```python
from build123d import *

# Parameters (mm, degrees)
F0_R     = 14.2875
F0_R_2   = 3.373438
F1_DEPTH = 2.286


with BuildPart() as f1:
    # F0 (on Front) → F1 (new body)
    with BuildSketch(Plane.XZ):
        with BuildLine():
            ThreePointArc((-34.573266, -67.66252), (-26.367008, -66.963304), (-18.815872, -63.675156))
            Line((-18.815872, -63.675156), (136.129614, 36.414264))
            ThreePointArc((136.129614, 36.414264), (146.710231, 64.934436), (122.34748, 83.14998))
            Line((122.34748, 83.14998), (37.837742, 83.14998))
            ThreePointArc((37.837742, 83.14998), (27.550148, 85.3266), (19.025718, 91.483412))
            Line((19.025718, 91.483412), (-13.74376, 116.798291))
            ThreePointArc((-13.74376, 116.798291), (-32.877689, 121.840327), (-49.823331, 111.623939))
            Line((-49.823331, 111.623939), (-138.293377, -10.186806))
            ThreePointArc((-138.293377, -10.186806), (-141.899369, -17.266125), (-143.141887, -25.113168))
            Line((-143.141887, -25.113168), (-143.141887, -42.26252))
            ThreePointArc((-143.141887, -42.26252), (-135.7024, -60.223032), (-117.741887, -67.66252))
            Line((-117.741887, -67.66252), (-34.573266, -67.66252))
        make_face()
        with Locations((-20.212744, -35.91252)):
            Circle(F0_R, mode=Mode.SUBTRACT)
        Polygon((-75.897325, -20.576264), (-88.5972, -20.519901), (-94.898326, -9.493306), (-88.499577, 1.476927), (-75.799702, 1.420565), (-69.498576, -9.606031), align=None, mode=Mode.SUBTRACT)
        Polygon((-75.839717, 7.770723), (-88.539592, 7.827085), (-94.840718, 18.853681), (-88.441969, 29.823914), (-75.742094, 29.767551), (-69.440968, 18.740956), align=None, mode=Mode.SUBTRACT)
        Polygon((-48.344767, -5.516115), (-61.044642, -5.459752), (-67.345768, 5.566844), (-60.947019, 16.537077), (-48.247144, 16.480714), (-41.946018, 5.454118), align=None, mode=Mode.SUBTRACT)
        Polygon((6.38129, -3.277528), (-6.318585, -3.221165), (-12.619711, 7.80543), (-6.220962, 18.775663), (6.478913, 18.719301), (12.780039, 7.692705), align=None, mode=Mode.SUBTRACT)
        Polygon((-19.443963, 11.747547), (-32.143838, 11.80391), (-38.444964, 22.830506), (-32.046215, 33.800739), (-19.34634, 33.744376), (-13.045214, 22.71778), align=None, mode=Mode.SUBTRACT)
        Polygon((31.725593, -16.542709), (19.025718, -16.486347), (12.724592, -5.459751), (19.123341, 5.510482), (31.823216, 5.454119), (38.124342, -5.572476), align=None, mode=Mode.SUBTRACT)
        Polygon((31.570362, 11.803911), (18.870487, 11.860274), (12.569361, 22.886869), (18.96811, 33.857102), (31.667985, 33.80074), (37.969111, 22.774144), align=None, mode=Mode.SUBTRACT)
        Polygon((57.344158, -3.27753), (44.644283, -3.221167), (38.343157, 7.805429), (44.741906, 18.775662), (57.441781, 18.719299), (63.742907, 7.692703), align=None, mode=Mode.SUBTRACT)
        Polygon((83.04678, 13.283836), (70.346906, 13.340383), (64.04594, 24.367071), (70.444848, 35.337211), (83.144723, 35.280663), (89.445688, 24.253976), align=None, mode=Mode.SUBTRACT)
        Polygon((-48.499998, 22.830506), (-61.199873, 22.886868), (-67.500999, 33.913464), (-61.10225, 44.883697), (-48.402375, 44.827334), (-42.101249, 33.800739), align=None, mode=Mode.SUBTRACT)
        Polygon((6.226059, 25.069092), (-6.473816, 25.125455), (-12.774942, 36.152051), (-6.376193, 47.122284), (6.323682, 47.065921), (12.624808, 36.039325), align=None, mode=Mode.SUBTRACT)
        Polygon((-48.44239, 51.177492), (-61.142265, 51.233855), (-67.443391, 62.260451), (-61.044642, 73.230684), (-48.344767, 73.174321), (-42.043641, 62.147725), align=None, mode=Mode.SUBTRACT)
        with Locations((-27.847204, 58.683684)):
            Circle(F0_R_2, mode=Mode.SUBTRACT)
        Polygon((6.283667, 53.416079), (-6.416208, 53.472442), (-12.717334, 64.499037), (-6.318585, 75.46927), (6.38129, 75.412908), (12.682416, 64.386312), align=None, mode=Mode.SUBTRACT)
        with Locations((-27.847204, 84.083684)):
            Circle(F0_R, mode=Mode.SUBTRACT)
        with Locations((-27.847204, 109.483684)):
            Circle(F0_R_2, mode=Mode.SUBTRACT)
        Polygon((57.188926, 25.06909), (44.489052, 25.125453), (38.187926, 36.152049), (44.586675, 47.122282), (57.28655, 47.065919), (63.587675, 36.039323), align=None, mode=Mode.SUBTRACT)
        Polygon((31.62797, 40.150898), (18.928095, 40.20726), (12.626969, 51.233856), (19.025718, 62.204089), (31.725593, 62.147726), (38.026719, 51.121131), align=None, mode=Mode.SUBTRACT)
        Polygon((57.246534, 53.416077), (44.54666, 53.47244), (38.245534, 64.499036), (44.644283, 75.469269), (57.344158, 75.412906), (63.645284, 64.38631), align=None, mode=Mode.SUBTRACT)
        with Locations((88.855389, 56.16248)):
            Circle(F0_R, mode=Mode.SUBTRACT)
        with Locations((124.415389, 56.16248)):
            Circle(F0_R, mode=Mode.SUBTRACT)
    extrude(amount=F1_DEPTH)


solid = f1.part
```
Build history of the part. All positions in model axes, mm. Round coordinates to 2 decimals unless told otherwise and drop trailing zeros. Write each loop counter-clockwise with the first axis right and the second up, starting at its lowest first coordinate (ties: lowest second). Pieces come first, ordered by that corner, then holes.
1) Band-saw the part on C-C, the plane y = -1.5. Give the number of separate pieces and of enclosed holes in the cut face, and give its area (3 significant figures).
2) Drill centre lines: probe 1 along Z at (x, y) = (-65, -1.05); probe 2 along X at (y, z) = (-1.95, 47); probe 3 along X at (y, z) = (-1.4, 19). Where is each one in solid material? Low to high.
3) Band-saw the part on B-B, the plane x = -56. List the corners of the cut face in (y, z), and give its area (3 significant figures).
4) Band-saw the part on A-A, the plane z = -30. List the corners of the cut face in (x, y), and give its area (3 significant figures).
5) Mould opens along X. For faces 1 (the flat face through (-32, -2.286, 7)), 2 (the flat face through (-9.62, -1.13, 41.56)), 3 (the flat face through (-93.44, -1.13, 51.57)) say: +X half, -X half, draft (parallel to the pull), parting line (faces both ways), or undercut.
6) Pin check, flat tips, straight feed: pin 1 (23 mm diameter, centred on x = 124.42, z = 56.16, fed in from +Y); pin 2 (0.7 mm diameter, centred on x = 87, y = -1.5, fed in from +Z). Stop position of each tip, or through.
Ans:
1. separate pieces: 1
1. enclosed holes: 22
1. area: 23,300 mm2
2. probe 1: z = -67.66 to 1.46, 9.59 to 29.54, 38.2 to 57.98, 66.45 to 90.73
2. probe 2: x = -96.76 to -6.45, 6.36 to 15.05, 35.62 to 44.52, 57.32 to 77.89, 99.82 to 113.45, 135.38 to 145.36
2. probe 3: x = -117.1 to -94.76, -69.59 to -36.26, -15.21 to 14.79, 35.77 to 67.11, 86.38 to 109.17
3. outline: (-2.29, -67.66) - (0, -67.66) - (0, -5.48) - (-2.29, -5.48) - close; (-2.29, 16.52) - (0, 16.52) - (0, 22.86) - (-2.29, 22.86) - close; (-2.29, 44.86) - (0, 44.86) - (0, 51.21) - (-2.29, 51.21) - close; (-2.29, 73.21) - (0, 73.21) - (0, 103.12) - (-2.29, 103.12) - close
3. area: 240 mm2
4. outline: (-143.14, -2.29) - (-33.22, -2.29) - (-33.22, 0) - (-143.14, 0) - close; (-7.21, -2.29) - (33.32, -2.29) - (33.32, 0) - (-7.21, 0) - close
4. area: 344 mm2
5. face 1: draft
5. face 2: undercut
5. face 3: -X half
6. pin 1: passes through
6. pin 2: stops at z = 83.15
